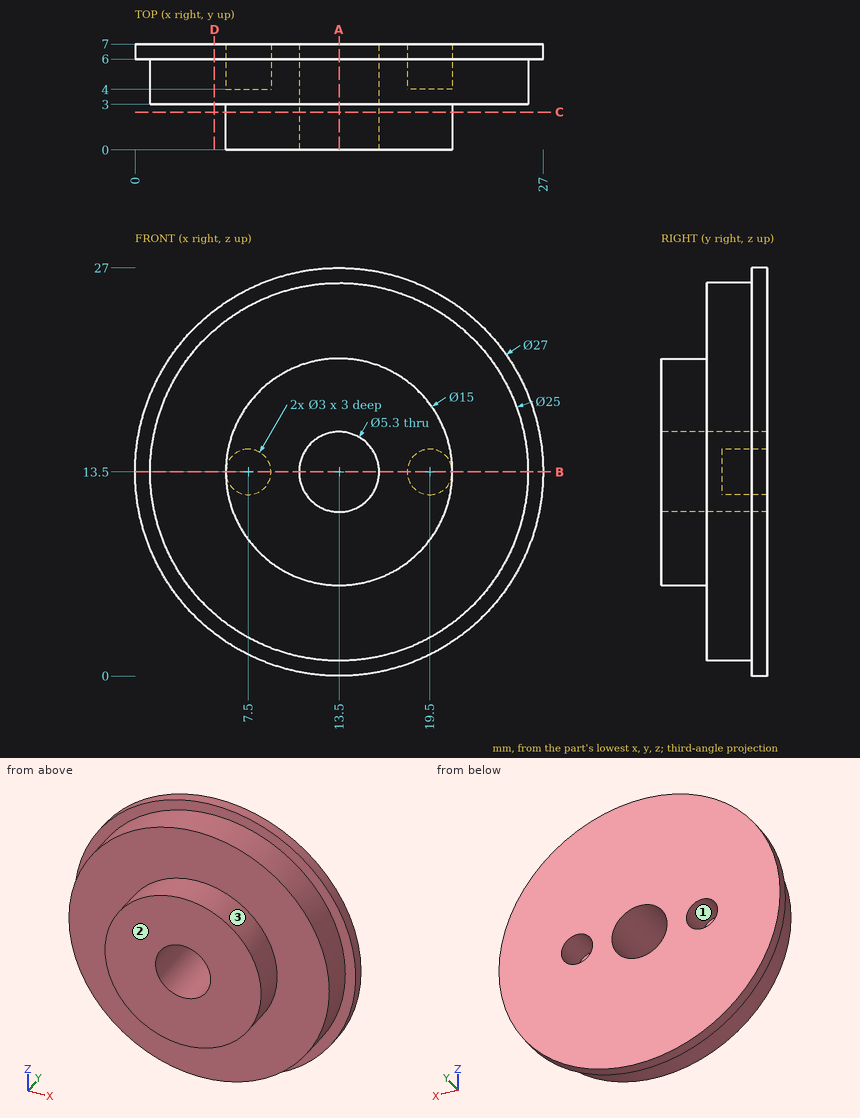
Study the drawing (mm; zero at the part's minimum x, y, z) and answer. A direction names the side the tool comes from. Give positions to 0.01 mm unless a question says otherwise; leave off trailing zeros. Order: outer loops, then holes, each group sorted by start corner. A loop starts at its lowest first (then second) coordinate and runs counter-clockwise, first axis right, second up. Notation, with made-up numbers: (8, 40) -> (33, 40) arc R32 ccw to (33, 69) -> close; hole circle Ø10 at (84.25, 14). An arc over 180 degrees is marked (long way). Put each result on its own line as item: value.
Item 1: A cutting plane is placed at B-B on z = 13.5. Give the vertices of the cut face in (x, y).
Established:
outline: (0, 6) -> (1, 6) -> (1, 3) -> (6, 3) -> (6, 0) -> (10.85, 0) -> (10.85, 7) -> (9, 7) -> (9, 4) -> (6, 4) -> (6, 7) -> (0, 7) -> close; (16.15, 0) -> (21, 0) -> (21, 3) -> (26, 3) -> (26, 6) -> (27, 6) -> (27, 7) -> (21, 7) -> (21, 4) -> (18, 4) -> (18, 7) -> (16.15, 7) -> close
Item 2: A cutting plane is placed at C-C on y = 2.5. Give the vertices of the cut face in (x, z).
Established:
outline: circle Ø15 at (13.5, 13.5); hole circle Ø5.3 at (13.5, 13.5)
Item 3: Straight lines are drawn through the part: line 1 (X direction, y = 5.5, z = 12.25); line 2 (Y direction, x = 23.25, z = 7.5); line 3 (Z direction, x = 7.5, y = 5.1). For each, find the intervals that lie inside material, in ascending order.
Established:
line 1: x = 1.06 to 6.67, 8.33 to 11.16, 15.84 to 18.67, 20.33 to 25.94
line 2: y = 3 to 7
line 3: z = 2.53 to 12, 15 to 24.47
Item 4: A cutting plane is placed at D-D on x = 5.25. Give the vertices of the cut face in (y, z).
Established:
outline: (3, 4.11) -> (6, 4.11) -> (6, 2.81) -> (7, 2.81) -> (7, 24.19) -> (6, 24.19) -> (6, 22.89) -> (3, 22.89) -> close
Item 5: Given P1, Ø3, axis at x = 20.5, y = 5.5, coming from the +Z side; P2, Ø4, axis at y = 2.5, z = 13, coming from the -X side; P3, Ø5, axis at x = 6.5, z = 3.5, coming from the -Y side, each flat-ended and moving along its own axis, determine where each tip first touches the part or whether it passes through.
Established:
P1: stops at z = 25.79
P2: stops at x = 1
P3: stops at y = 3
Item 6: For the marked faces 1, 2 and 3, determine the directions among +Z, -Z, +X, -X, +Y, -Y from which every point of the face is accessible in a straight line to the end or side of a thin tool.
Established:
face 1: +Y
face 2: +Z, -Z, +X, -X, -Y
face 3: -Y
Item 7: A cutting plane is placed at A-A on x = 13.5. Give the vertices of the cut face in (y, z).
Established:
outline: (0, 6) -> (3, 6) -> (3, 1) -> (6, 1) -> (6, 0) -> (7, 0) -> (7, 10.85) -> (0, 10.85) -> close; (0, 16.15) -> (7, 16.15) -> (7, 27) -> (6, 27) -> (6, 26) -> (3, 26) -> (3, 21) -> (0, 21) -> close
